```python
from build123d import *

# Parameters (mm, degrees)
PAD_DEPTH       = 13
POCKET_DEPTH    = 10
SKETCH003_R     = 1.85
PAD001_DEPTH    = 7
FILLET_R        = 1
POCKET001_DEPTH = 5


with BuildPart() as part:
    # Sketch → Pad (new body)
    with BuildSketch(Plane.XY):
        Polygon((7.85, 4.1), (-5.010546, 4.1), (-7.85, 1.5), (-7.85, -1.5), (-5.010546, -4.1), (7.85, -4.1), align=None)
    extrude(amount=PAD_DEPTH)

    # Sketch002 → Pocket (cut)
    with BuildSketch(Plane.XY.offset(16)):
        Polygon((7.5, 4), (-4.825509, 4), (-7.5, 1.4), (-7.5, -1.4), (-4.825509, -4), (7.5, -4), align=None)
    extrude(amount=-POCKET_DEPTH, mode=Mode.SUBTRACT)

    # Sketch003 (on Face15 of Pocket) → Pad001 (join)
    with BuildSketch(Plane.XY.offset(6)):
        with Locations((-3.6, 0)):
            Circle(SKETCH003_R)
        with Locations((3.6, 0)):
            Circle(SKETCH003_R)
    extrude(amount=PAD001_DEPTH)

    # Fillet
    fillet_edges = [part.edges().sort_by_distance(p)[0] for p in [
        (-5.45, 0, 13),
        (1.75, 0, 13),
    ]]
    fillet(fillet_edges, radius=FILLET_R)

    # Sketch004 (on Face4 of Fillet) → Pocket001 (cut)
    with BuildSketch(Plane.XY.offset(13)):
        Polygon((-3.85, 2.25), (-3.35, 2.25), (-3.35, 0.25), (-1.35, 0.25), (-1.35, -0.25), (-3.35, -0.25), (-3.35, -2.25), (-3.85, -2.25), (-3.85, -0.25), (-5.85, -0.25), (-5.85, 0.25), (-3.85, 0.25), align=None)
        Polygon((3.85, 2.25), (3.35, 2.25), (3.35, 0.25), (1.35, 0.25), (1.35, -0.25), (3.35, -0.25), (3.35, -2.25), (3.85, -2.25), (3.85, -0.25), (5.85, -0.25), (5.85, 0.25), (3.85, 0.25), align=None)
    extrude(amount=-POCKET001_DEPTH, mode=Mode.SUBTRACT)


solid = part.part
```
The model under review builds one solid part; all positions refer to its coordinate system, in mm. A direction names the side the tool comes from. Give positions to 0.01 mm unless a question says otherwise; leave off trailing zeros. Write each loop counter-clockwise with the first axis right and the second up, starting at its lowest first coordinate (ties: lowest second). Pieces come first, ordered by that corner, then holes. Notation, with made-up numbers: (34.25, 79) -> (91.25, 79) arc R12 cw to (91.25, 85) -> close; hole circle Ø2 at (30.5, -20.5). An arc over 180 degrees is marked (long way). Put each result on its own line as item: value.
(1) We need section B-B, the plane y = 0. Give the boundary of the cut face in (x, z), and give its area (3 significant figures).
Results are:
outline: (-7.85, 0) -> (7.85, 0) -> (7.85, 13) -> (7.5, 13) -> (7.5, 6) -> (5.45, 6) -> (5.45, 8) -> (1.75, 8) -> (1.75, 6) -> (-1.75, 6) -> (-1.75, 8) -> (-5.45, 8) -> (-5.45, 6) -> (-7.5, 6) -> (-7.5, 13) -> (-7.85, 13) -> close
area: 114 mm²
(2) To check wall thickness, follow probe 1 along X at (y, z) = (0.75, 9); probe 2 along Z at (x, y) = (-2.5, -1.75); probe 3 along X at (y, z) = (1.25, 8.75). State the ranges of each line that lie inside material, in increasing order. Write a range as from..to.
Results are:
probe 1: -7.85..-7.5, -5.29..-3.85, -3.35..-1.91, 1.91..3.35, 3.85..5.29, 7.5..7.85
probe 2: 0..6
probe 3: -7.85..-7.5, -4.96..-3.85, -3.35..-2.24, 2.24..3.35, 3.85..4.96, 7.5..7.85
(3) Tool access review of faces 1 (the flat face through (-4, 0, 8)), 2 (the flat face through (0, 0, 0)): name each direction out of +Z, -Z, +X, -X, +Y, -Y from which nothing blocks a thin tool from reaching the whole face with its end or side.
Results are:
face 1: +Z
face 2: -Z, +X, -X, +Y, -Y
(4) We need section D-D, the plane z = 9.25. State how many separate pieces and enclosed holes the cut face has, and give its area (3 significant figures).
Results are:
separate pieces: 9
enclosed holes: 1
area: 22.9 mm²
(5) We need section C-C, the plane x = 3.6. Give the boundary of the cut face in (y, z), and give its area (3 significant figures).
Results are:
outline: (-4.1, 0) -> (4.1, 0) -> (4.1, 13) -> (4, 13) -> (4, 6) -> (1.85, 6) -> (1.85, 8) -> (-1.85, 8) -> (-1.85, 6) -> (-4, 6) -> (-4, 13) -> (-4.1, 13) -> close
area: 58.0 mm²
(6) We need section A-A, the plane z = 6.5. Give the boundary of the cut face in (x, y), and give its area (3 significant figures).
Results are:
outline: (-7.85, -1.5) -> (-5.01, -4.1) -> (7.85, -4.1) -> (7.85, 4.1) -> (-5.01, 4.1) -> (-7.85, 1.5) -> close; circle Ø3.7 at (-3.6, 0); circle Ø3.7 at (3.6, 0); hole (-7.5, -1.4) -> (-4.83, -4) -> (7.5, -4) -> (7.5, 4) -> (-4.83, 4) -> (-7.5, 1.4) -> close
area: 29.8 mm²
(7) The part is to be moulded in two halves that separate along X. For faces 3 (the flat face through (2, 4.1, 5)), 4 (the flat face through (7.85, 0, 6)), 5 (the flat face through (0, 0, 6)), say which applies: pulls with the +X half, pulls with the -X half, needs draft (parallel to the pull), parting line crosses it, or undercut.
Results are:
face 3: needs draft
face 4: pulls with the +X half
face 5: undercut
